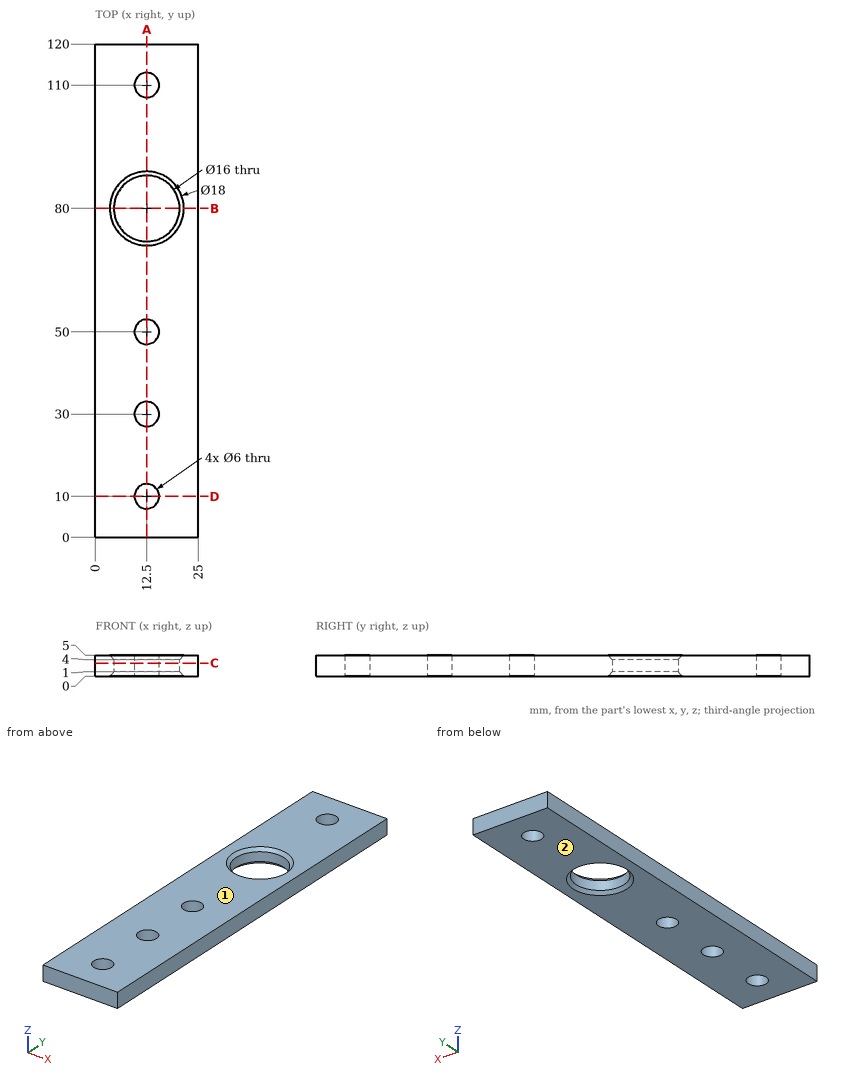
Part print with two shaded views. Sizes in mm from the minimum x, y, z corner. Coordinates: 2 decimals unless noted, no trailing zeros. Write each loop counter-clockwise with the first axis right and the second up, starting at its lowest first coordinate (ties: lowest second). Pieces come first, ordered by that corner, then holes. Notation, with made-up numbers: (-4.75, -23) - (48.25, -23) arc R14 cw to (48.25, -12) - close; hole circle Ø1 at (-10, -10). An arc over 180 degrees is marked (long way). Use a Markdown table: item, result. Add a question column.
Item 1: Band-saw the part on D-D, the plane y = 10. Write the cut outline in (x, z), and give its area (3 significant figures).
Item 2: Drill centre lines: line 1 along Y through (x, z) = (12.5, 2.35); line 2 along Y through (x, z) = (11.25, 2.3); line 3 along X through (y, z) = (31, 0.7). Where is each one in solid material? Low to high.
Item 3: Band-saw the part on A-A, the plane x = 12.5. Write the cut outline in (y, z).
Item 4: Band-saw the part on B-B, the plane y = 80. Write the cut outline in (x, z).
Item 5: Drop a flat-ended pin along its axis: pin 1 (1 mm diameter, centred on x = 5.5, z = 3.5, fed in from -Y). Give the stop position or say it passes through.
Item 6: Band-saw the part on C-C, the plane z = 3.15. Write the cut outline in (x, y).
Item 7: Two-plate mould, pull along Z, no slides. Class the marked faces 1 and 2: pulls with the +Z half, pulls with the -Z half, needs draft (parallel to the pull), parting line crosses it, or undercut.
A:
| question | item | result |
|---|---|---|
| 1 | outline | (0, 0) - (9.5, 0) - (9.5, 5) - (0, 5) - close; (15.5, 0) - (25, 0) - (25, 5) - (15.5, 5) - close |
| 1 | area | 95.0 mm² |
| 2 | line 1 | y = 0 to 7, 13 to 27, 33 to 47, 53 to 72, 88 to 107, 113 to 120 |
| 2 | line 2 | y = 0 to 7.27, 12.73 to 27.27, 32.73 to 47.27, 52.73 to 72.1, 87.9 to 107.27, 112.73 to 120 |
| 2 | line 3 | x = 0 to 9.67, 15.33 to 25 |
| 3 | outline | (0, 0) - (7, 0) - (7, 5) - (0, 5) - close; (13, 0) - (27, 0) - (27, 5) - (13, 5) - close; (33, 0) - (47, 0) - (47, 5) - (33, 5) - close; (53, 0) - (71, 0) - (72, 1) - (72, 4) - (71, 5) - (53, 5) - close; (88, 1) - (89, 0) - (107, 0) - (107, 5) - (89, 5) - (88, 4) - close; (113, 0) - (120, 0) - (120, 5) - (113, 5) - close |
| 4 | outline | (0, 0) - (3.5, 0) - (4.5, 1) - (4.5, 4) - (3.5, 5) - (0, 5) - close; (20.5, 1) - (21.5, 0) - (25, 0) - (25, 5) - (21.5, 5) - (20.5, 4) - close |
| 5 | pin 1 | stops at y = 0 |
| 6 | outline | (0, 0) - (25, 0) - (25, 120) - (0, 120) - close; hole circle Ø16 at (12.5, 80); hole circle Ø6 at (12.5, 10); hole circle Ø6 at (12.5, 30); hole circle Ø6 at (12.5, 50); hole circle Ø6 at (12.5, 110) |
| 7 | face 1 | pulls with the +Z half |
| 7 | face 2 | pulls with the -Z half |
